from build123d import *
from OCP.BRepAlgoAPI import BRepAlgoAPI_Cut
from OCP.TopTools import TopTools_ListOfShape

# Parameters (mm, degrees)
SKETCH1_W            = 18.581245514
SKETCH1_H            = 1.5
SKETCH2_R            = 7.5
CUT_EXTRUDE1_DEPTH   = 24.5
SHELL1_OUTLINE_R     = 18.581245514
SHELL1_DEPTH         = 27.672789125
SHELL1_START         = 27.672789125
SHELL1_2_OUTLINE_R   = 15.581245514
SHELL1_2_DEPTH       = 9.327210875
SHELL1_START_2       = 35.172789125
SHELL1_3_OUTLINE_R   = 18.581245514
SHELL1_3_OUTLINE_R_2 = 15.581245514
SHELL1_3_DEPTH       = 1.827210875
SHELL1_START_3       = -18.581245614
SHELL1_4_OUTLINE_R   = 10.5
SHELL1_4_OUTLINE_R_2 = 7.5
SHELL1_4_DEPTH       = 37.162490158
SKETCH3_W            = 25
SKETCH3_H            = 25
CUT_EXTRUDE2_DEPTH   = 7.5


with BuildPart() as part:
    # Sketch1 → Revolve1 (revolve)
    with BuildSketch(Plane.XY, mode=Mode.PRIVATE) as revolve1_sk:
        with BuildLine():
            Line((0, 40), (0, 36.972789125))
            Line((0, 36.972789125), (21.581245514, 36.972789125))
            ThreePointArc((21.581245514, 36.972789125), (10.896262703, 39.239510786), (0, 40))
        make_face()
        Polygon((0, 36.972789125), (0, 35.172789125), (18.581245514, 35.172789125), (21.581245514, 35.172789125), (21.581245514, 36.972789125), align=None)
        with Locations((9.290622757, 34.422789125)):
            Rectangle(SKETCH1_W, SKETCH1_H)
        Polygon((0, 33.672789125), (0, 32.172789125), (18.581245514, 32.172789125), (21.581245514, 32.172789125), (21.581245514, 33.672789125), (18.581245514, 33.672789125), align=None)
        with Locations((9.290622757, 31.422789125)):
            Rectangle(SKETCH1_W, SKETCH1_H)
        Polygon((0, 30.672789125), (0, 0), (21.581245514, 0), (21.581245514, 30.672789125), (18.581245514, 30.672789125), align=None)
    revolve(revolve1_sk.sketch.rotate(Axis((0, 0, 0), (0, 1, 0)), 90), axis=Axis((0, 0, 0), (0, 1, 0)))

    # Sketch2 → Cut-Extrude1 (cut, symmetric)
    with BuildSketch(Plane.XY):
        with Locations((0, 15.336394563)):
            Circle(SKETCH2_R)
    extrude(amount=CUT_EXTRUDE1_DEPTH, both=True, mode=Mode.SUBTRACT)


with BuildPart() as shell1_tool:
    # Shell1: read off the stored shape, not the designer's step
    # Shell1 outline → Shell1 (new body)
    with BuildSketch(Plane(origin=(0, 0, 0), x_dir=(1, 0, 0), z_dir=(0, 1, 0))):
        Circle(SHELL1_OUTLINE_R)
    extrude(amount=SHELL1_DEPTH)


with BuildPart() as part_1:
    add(part.part)

    # Shell1: cut by shell1_tool, with a tolerance
    shell1_stock = TopTools_ListOfShape()
    shell1_stock.Append(part_1.part.wrapped)
    shell1_tools = TopTools_ListOfShape()
    shell1_tools.Append(shell1_tool.part.wrapped)
    shell1_cut = BRepAlgoAPI_Cut()
    shell1_cut.SetArguments(shell1_stock)
    shell1_cut.SetTools(shell1_tools)
    shell1_cut.SetFuzzyValue(0.00001)
    shell1_cut.Build()
    add(Compound.cast(shell1_cut.Shape()).solids(), mode=Mode.REPLACE)


with BuildPart() as shell1_2_tool:
    # Shell1 2 outline → Shell1 2 (new body)
    with BuildSketch(Plane(origin=(0, 0, 0), x_dir=(1, 0, 0), z_dir=(0, 1, 0)).offset(SHELL1_START)):
        Circle(SHELL1_2_OUTLINE_R)
    extrude(amount=SHELL1_2_DEPTH)


with BuildPart() as part_2:
    add(part_1.part)

    # Shell1 2: cut by shell1_2_tool, with a tolerance
    shell1_2_stock = TopTools_ListOfShape()
    shell1_2_stock.Append(part_2.part.wrapped)
    shell1_2_tools = TopTools_ListOfShape()
    shell1_2_tools.Append(shell1_2_tool.part.wrapped)
    shell1_2_cut = BRepAlgoAPI_Cut()
    shell1_2_cut.SetArguments(shell1_2_stock)
    shell1_2_cut.SetTools(shell1_2_tools)
    shell1_2_cut.SetFuzzyValue(0.00001)
    shell1_2_cut.Build()
    add(Compound.cast(shell1_2_cut.Shape()).solids(), mode=Mode.REPLACE)


with BuildPart() as shell1_3_tool:
    # Shell1 3 outline → Shell1 3 (new body)
    with BuildSketch(Plane(origin=(0, 0, 0), x_dir=(1, 0, 0), z_dir=(0, 1, 0)).offset(SHELL1_START_2)):
        Circle(SHELL1_3_OUTLINE_R)
        Circle(SHELL1_3_OUTLINE_R_2, mode=Mode.SUBTRACT)
    extrude(amount=SHELL1_3_DEPTH)


with BuildPart() as part_3:
    add(part_2.part)

    # Shell1 3: cut by shell1_3_tool, with a tolerance
    shell1_3_stock = TopTools_ListOfShape()
    shell1_3_stock.Append(part_3.part.wrapped)
    shell1_3_tools = TopTools_ListOfShape()
    shell1_3_tools.Append(shell1_3_tool.part.wrapped)
    shell1_3_cut = BRepAlgoAPI_Cut()
    shell1_3_cut.SetArguments(shell1_3_stock)
    shell1_3_cut.SetTools(shell1_3_tools)
    shell1_3_cut.SetFuzzyValue(0.00001)
    shell1_3_cut.Build()
    add(Compound.cast(shell1_3_cut.Shape()).solids(), mode=Mode.REPLACE)


with BuildPart() as shell1_4_tool:
    # Shell1 4 outline → Shell1 4 (new body)
    with BuildSketch(Plane.XY.offset(SHELL1_START_3)):
        with Locations((0, 15.336394563)):
            Circle(SHELL1_4_OUTLINE_R)
        with Locations((0, 15.336394563)):
            Circle(SHELL1_4_OUTLINE_R_2, mode=Mode.SUBTRACT)
    extrude(amount=SHELL1_4_DEPTH)


with BuildPart() as part_4:
    add(part_3.part)


with BuildPart() as part_5:
    # Shell1 4: joined with shell1_4_tool
    add(part_4.part.fuse(shell1_4_tool.part, tol=0.00001))


with BuildPart() as shell1_5_tool:
    # Shell1 5 outline → Shell1 5 (revolve)
    with BuildSketch(Plane.XY):
        with BuildLine():
            Line((18.581245514, 37), (0, 37))
            ThreePointArc((0, 37), (8.301999629, 36.541805844), (16.503153993, 35.172789109))
            Line((16.503153993, 35.172789109), (18.581245514, 35.172789109))
            Line((18.581245514, 35.172789109), (18.581245514, 37))
        make_face()
    revolve(axis=Axis((0, 0, 0), (0, 1, 0)))


with BuildPart() as part_6:
    add(part_5.part)


with BuildPart() as part_7:
    # Shell1 5: joined with shell1_5_tool
    add(part_6.part.fuse(shell1_5_tool.part, tol=0.00001))

    # Sketch3 → Cut-Extrude2 (cut, symmetric)
    with BuildSketch(Plane.XY):
        with Locations((0, 15.336394563)):
            Rectangle(SKETCH3_W, SKETCH3_H)
    extrude(amount=CUT_EXTRUDE2_DEPTH, both=True, mode=Mode.SUBTRACT)


solid = part_7.part
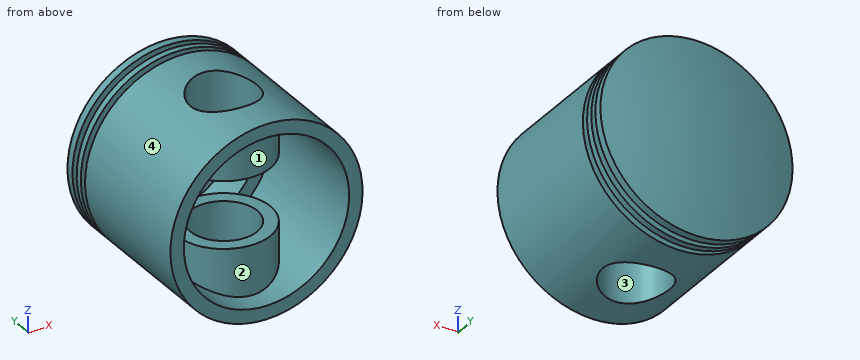
Could you check a few things on this model? Use its own coordinates, in mm. Face numbers are marked on the shaded views. Coordinates: 2 decimals unless noted, no trailing zeros. Order: outer loops, then holes, each group sorted by start corner. A loop starts at its lowest first (then second) coordinate and runs counter-clockwise, first axis right, second up. Notation, with made-up numbers: (-7.75, -29.5) - (2.25, -29.5) arc R24 cw to (2.25, -5.5) - close; hole circle Ø2 at (4, -13.75). An arc over 180 degrees is marked (long way). Answer in a Markdown table with one row per item. Add a question column.
(1) If we section it at A-A, the plane z = -10: State how many separate pieces and enclosed holes the cut face has, then the cut area to 3 significant figures.
(2) Will these pins go through, and if not, where does the flat tip stop? pin 1 (13 mm diameter, centred on x = 4.5, z = 0.5, fed in from -Y); pin 2 (10 mm diameter, centred on x = 4.5, z = 3, fed in from +Y); pin 3 (25 mm diameter, centred on x = 0, z = 0, fed in from -Y).
(3) If we mould it in two halves opening along Z, with no side actions, what happens to the marked faces 1, 2, 3 and 4? For each: released by +Z, released by -Z, zero draft, split by the parting line, or undercut.
(4) I need wall thicknesses on L1, parallel to X at y = 33, z = 0; L2, parallel to Y at x = 0, z = 13; L3, parallel to Z at x = -0.5, y = 24.5. Which ranges of each line are inside material? Lowest first, please.
(5) If we section it at D-D, the plane y = 12: Please give me the cut outline in (x, z).
(6) If we section it at C-C, the plane y = 7: Please give me the cut outline in (x, z).
Results are:
| question | item | result |
|---|---|---|
| 1 | separate pieces | 2 |
| 1 | enclosed holes | 1 |
| 1 | area | 558 mm2 |
| 2 | pin 1 | stops at y = 36.19 |
| 2 | pin 2 | stops at y = 40 |
| 2 | pin 3 | stops at y = 4.84 |
| 3 | face 1 | undercut |
| 3 | face 2 | undercut |
| 3 | face 3 | zero draft |
| 3 | face 4 | split by the parting line |
| 4 | L1 | x = -21.58 to -15.58, 15.58 to 21.58 |
| 4 | L2 | y = 4.84 to 7.84, 22.84 to 25.84, 35.87 to 38.92 |
| 4 | L3 | z = -21.58 to -7.5, 7.5 to 21.58 |
| 5 | outline | (-9.96, -15.69) arc R18.58 cw to (-9.96, 15.69) - (-9.96, 7.5) - (-6.72, 7.5) - (-6.72, 20.51) arc R21.58 ccw to (-6.72, -20.51) - (-6.72, -7.5) - (-9.96, -7.5) - close; (6.72, -20.51) arc R21.58 ccw to (6.72, 20.51) - (6.72, 7.5) - (9.96, 7.5) - (9.96, 15.69) arc R18.58 cw to (9.96, -15.69) - (9.96, -7.5) - (6.72, -7.5) - close |
| 6 | outline | circle Ø43.16 at (0, 0); hole (-6.38, -17.45) - (-6.38, -7.5) - (6.38, -7.5) - (6.38, -17.45) arc R18.58 ccw to (6.38, 17.45) - (6.38, 7.5) - (-6.38, 7.5) - (-6.38, 17.45) arc R18.58 ccw to start |
